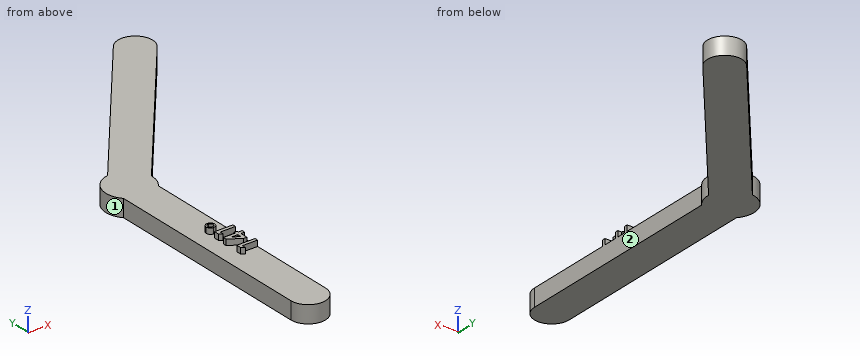
```python
from build123d import *

# Parameters (mm, degrees)
BOSS_EXTRUDE1_DEPTH = 3
BOSS_EXTRUDE2_DEPTH = 1


with BuildPart() as part:
    # Sketch2 → Boss-Extrude1 (new body)
    with BuildSketch(Plane.XY):
        with BuildLine():
            Line((-3, -40), (-3, -2.645751311))
            ThreePointArc((-3, -2.645751311), (-3.770565964, 1.335227437), (-0.666412635, 3.94409612))
            Line((-0.666412635, 3.94409612), (22.841377758, 32.973799631))
            ThreePointArc((22.841377758, 32.973799631), (27.060776815, 33.417276343), (27.504253526, 29.197877285))
            Line((27.504253526, 29.197877285), (3.996463134, 0.168173773))
            ThreePointArc((3.996463134, 0.168173773), (3.770565964, -1.335227437), (3, -2.645751311))
            Line((3, -2.645751311), (3, -40))
            ThreePointArc((3, -40), (0, -43), (-3, -40))
        make_face()
    extrude(amount=BOSS_EXTRUDE1_DEPTH)

    # Sketch3 → Boss-Extrude2 (add)
    # profile 1 of 4: a face of its own
    with BuildSketch(Plane.XY.offset(3)):
        Polygon((-0.175, -25.154881865), (-0.175, -24.27399745), (3, -24.27399745), (3, -24.843869245), (0.354166667, -24.843869245), (0.354166667, -25.495151297), align=None)
    # profile 2 of 4: a face of its own
    with BuildSketch(Plane.XY.offset(3)):
        Polygon((-0.256410256, -21.977973813), (-0.256410256, -21.383933348), (1.819551282, -21.383933348), (1.819551282, -21.09899745), (2.348717949, -21.09899745), (2.348717949, -21.383933348), (3, -21.383933348), (3, -21.953805143), (2.348717949, -21.953805143), (2.348717949, -23.297074373), (1.77184996, -23.297074373), align=None)
        Polygon((1.819551282, -21.953805143), (0.738957332, -21.953805143), (1.819551282, -22.656604622), align=None, mode=Mode.SUBTRACT)
    # profile 3 of 4: a face of its own
    with BuildSketch(Plane.XY.offset(3)):
        Polygon((-0.175, -20.188856224), (-0.175, -19.307971809), (3, -19.307971809), (3, -19.877843604), (0.354166667, -19.877843604), (0.354166667, -20.529125656), align=None)
    # profile 4 of 4: a face of its own
    with BuildSketch(Plane.XY.offset(3)):
        with BuildLine():
            add(Edge.make_bspline(
                [(0.476282051, -16.824958989), (0.501543872, -16.825505484), (0.55122174, -16.826580176), (0.624352745, -16.837013476), (0.694208258, -16.854492691), (0.761803607, -16.876903338), (0.825395964, -16.908042089), (0.886396731, -16.944903837), (0.943669883, -16.989402672), (0.9978957, -17.039014969), (1.047295391, -17.093515132), (1.090947065, -17.151405488), (1.127096601, -17.212864468), (1.157366856, -17.276577248), (1.180332148, -17.343408663), (1.196689885, -17.412864586), (1.20741609, -17.485236986), (1.208449037, -17.534503871), (1.208974359, -17.559559349)],
                knots=[0, 0, 0, 0, 1.048753193, 2.062393874, 3.059725798, 4.03711221, 5.013824111, 5.993903926, 6.992478922, 8.020738441, 9.043061753, 10.043343452, 11.026424807, 11.999358773, 12.968420071, 13.955122655, 14.960044262, 16, 16, 16, 16], degree=3))
            add(Edge.make_bspline(
                [(1.208974359, -17.559559349), (1.208454225, -17.584616682), (1.207431478, -17.633887214), (1.196631189, -17.706233128), (1.180530583, -17.775855144), (1.156529218, -17.842391691), (1.126678292, -17.90615653), (1.090260147, -17.967072817), (1.046482503, -18.024600993), (0.996781055, -18.078582797), (0.942375086, -18.128107638), (0.88420218, -18.171482912), (0.823225465, -18.208946116), (0.758107997, -18.237837437), (0.69067286, -18.261947038), (0.619758864, -18.27798784), (0.545943315, -18.288833106), (0.495615647, -18.289833085), (0.469921875, -18.290343604)],
                knots=[0, 0, 0, 0, 1.037227242, 2.039512271, 3.023626077, 3.993053151, 4.963434463, 5.936395473, 6.927031705, 7.952593414, 8.972234493, 9.969891786, 10.954906455, 11.929570282, 12.915563215, 13.916770353, 14.936449251, 16, 16, 16, 16], degree=3))
            add(Edge.make_bspline(
                [(0.469921875, -18.290343604), (0.445290866, -18.289811451), (0.396869022, -18.288765297), (0.325492116, -18.278103661), (0.256787066, -18.261182775), (0.190979117, -18.23681523), (0.128167681, -18.205730248), (0.067236284, -18.169180135), (0.010175979, -18.123937412), (-0.044275745, -18.073515722), (-0.093962638, -18.018218509), (-0.137555056, -17.95952238), (-0.173973759, -17.89802202), (-0.203993097, -17.834134423), (-0.227847104, -17.767768562), (-0.244158222, -17.698411219), (-0.254789074, -17.626671533), (-0.255866772, -17.577830012), (-0.256410256, -17.553199173)],
                knots=[0, 0, 0, 0, 1.027628768, 2.020204677, 3.0054932, 3.977172113, 4.942988595, 5.928118098, 6.937247537, 7.976812879, 9.023474825, 10.036014018, 11.024160528, 12.002107364, 12.979092523, 13.962271943, 14.972371232, 16, 16, 16, 16], degree=3))
            add(Edge.make_bspline(
                [(-0.256410256, -17.553199173), (-0.255881051, -17.528566172), (-0.254836181, -17.479930408), (-0.244068832, -17.408427146), (-0.227959354, -17.339440503), (-0.203981879, -17.27352423), (-0.173948227, -17.210285117), (-0.137706982, -17.149501332), (-0.093944483, -17.091941849), (-0.043999627, -17.038019265), (0.009956511, -16.987787182), (0.068273488, -16.944627592), (0.128824771, -16.907104674), (0.192846684, -16.877455064), (0.259342082, -16.853394895), (0.329176204, -16.837233977), (0.401748506, -16.826543556), (0.451226198, -16.825491671), (0.476282051, -16.824958989)],
                knots=[0, 0, 0, 0, 1.02774298, 2.029191086, 3.012479778, 3.981238486, 4.951290381, 5.931946007, 6.930416638, 7.964088953, 8.997761269, 10.003308488, 10.98854748, 11.966603007, 12.943696749, 13.935593372, 14.954569896, 16, 16, 16, 16], degree=3))
        make_face()
        with BuildLine():
            add(Edge.make_bspline(
                [(0.479462139, -17.069189758), (0.462471258, -17.069424264), (0.428972226, -17.069886612), (0.379883793, -17.077505977), (0.332524379, -17.088023775), (0.287283463, -17.10328392), (0.24427911, -17.123234284), (0.203398935, -17.147571829), (0.164484674, -17.176174899), (0.128492582, -17.209237523), (0.095853701, -17.245103846), (0.066652511, -17.282897251), (0.042455186, -17.323086522), (0.023016589, -17.365273093), (0.006315159, -17.408801858), (-0.003707976, -17.454711924), (-0.01154919, -17.502263298), (-0.011966436, -17.534718897), (-0.012179487, -17.55129112)],
                knots=[0, 0, 0, 0, 1.061159961, 2.092171217, 3.098605391, 4.092036902, 5.070589041, 6.057187883, 7.061962211, 8.084674938, 9.107387665, 10.090954379, 11.06617917, 12.032717429, 12.99305519, 13.973669989, 14.965331307, 16, 16, 16, 16], degree=3))
            add(Edge.make_bspline(
                [(-0.012179487, -17.55129112), (-0.01157068, -17.568051412), (-0.01036426, -17.601263796), (-0.004409395, -17.650200831), (0.007572839, -17.69685371), (0.022606002, -17.742054962), (0.043122897, -17.784898142), (0.067542797, -17.826391236), (0.096744971, -17.865435361), (0.129769422, -17.902214665), (0.165718261, -17.935960463), (0.204573602, -17.964950546), (0.244977971, -17.990352408), (0.287582445, -18.010455361), (0.331832846, -18.026567734), (0.377821945, -18.038209426), (0.425871214, -18.044356322), (0.458458137, -18.045521173), (0.475010016, -18.046112835)],
                knots=[0, 0, 0, 0, 1.042034071, 2.064906527, 3.055369705, 4.030203466, 5.020228521, 6.000742353, 7.017744738, 8.043920206, 9.069249762, 10.075703201, 11.051782302, 12.029903876, 12.99669358, 13.974371501, 14.971122288, 16, 16, 16, 16], degree=3))
            add(Edge.make_bspline(
                [(0.475010016, -18.046112835), (0.491349767, -18.045520146), (0.523514051, -18.044353455), (0.570936909, -18.038223162), (0.616468237, -18.026465839), (0.660506807, -18.010425399), (0.703332854, -17.990458383), (0.743356347, -17.964229259), (0.782721478, -17.935019181), (0.819574977, -17.900938323), (0.853594861, -17.864058718), (0.883277913, -17.824563201), (0.908722399, -17.783622403), (0.929101491, -17.740636346), (0.945194342, -17.696373754), (0.956841315, -17.650387952), (0.962986781, -17.60233779), (0.964151827, -17.56975099), (0.96474359, -17.553199173)],
                knots=[0, 0, 0, 0, 1.017878107, 2.003660885, 2.970612419, 3.939454555, 4.919652619, 5.904816436, 6.913406512, 7.969270601, 9.02513469, 10.033724766, 11.041277553, 12.021475617, 12.990317753, 13.970071221, 14.968938047, 16, 16, 16, 16], degree=3))
            add(Edge.make_bspline(
                [(0.96474359, -17.553199173), (0.964515736, -17.536840687), (0.964066668, -17.504600367), (0.956359019, -17.457448889), (0.946146284, -17.411789288), (0.929505189, -17.368485652), (0.910263551, -17.326033898), (0.884925795, -17.286252494), (0.856415485, -17.247396305), (0.822504018, -17.212069657), (0.787116244, -17.177952839), (0.747777121, -17.149765554), (0.707718654, -17.124520148), (0.665616684, -17.10387006), (0.621397497, -17.089062601), (0.575848465, -17.07693948), (0.528165265, -17.071009446), (0.49579822, -17.069800121), (0.479462139, -17.069189758)],
                knots=[0, 0, 0, 0, 1.029744634, 2.029484694, 3.00508751, 3.97324883, 4.947661161, 5.937798898, 6.940036528, 7.980134083, 9.020231638, 10.033191535, 11.023329272, 12.003497406, 12.979740652, 13.958541426, 14.969648588, 16, 16, 16, 16], degree=3))
        make_face(mode=Mode.SUBTRACT)
    extrude(amount=BOSS_EXTRUDE2_DEPTH)


solid = part.part
```
The model under review builds one solid part; all positions refer to its coordinate system, in mm. Face numbers are marked on the shaded views. A direction names the side the tool comes from. Coordinates: 2 decimals unless noted, no trailing zeros. Write each loop counter-clockwise with the first axis right and the second up, starting at its lowest first coordinate (ties: lowest second). Pieces come first, ordered by that corner, then holes.
1) Clearance check with flat-ended pins moving along their axes: pin 1 Ø2 at (y, z) = (-18, 1.5) entering from +X; pin 2 Ø1 at (y, z) = (4.5, 3) entering from +X; pin 3 Ø10 at (x, y) = (6.5, 13) entering from -Z; pin 4 Ø0.8 at (x, z) = (1.5, 3.5) entering from -Y. State where each tip first meets the part, or that it passes through.
2) We need section B-B on y = -28. State the section outline as (x, z) points, then the cut area to 3 significant figures.
3) We need section A-A on z = 0.95. State the section outline as (x, y) points, then the cut area to 3 significant figures.
4) Machinability: for the marked faces 1 and 2, which of the approach directions +Z, -Z, +X, -X, +Y, -Y give a long, thin tool a straight path to every point of the face, cutting with its end or side? Answer none if there is none.
5) We need section C-C on x = 5. State the section outline as (y, z) points, then the cut area to 3 significant figures.
6) To check wall thickness, follow probe 1 along X at (y, z) = (-30, 1.3); probe 2 along Z at (x, y) = (11.5, 15.5); probe 3 along X at (y, z) = (15.5, 0.45). State the ranges of each line that lie inside material, in increasing order.
Answer list:
1. pin 1: stops at x = 3
1. pin 2: stops at x = 7.91
1. pin 3: stops at z = 0
1. pin 4: stops at y = -24.84
2. outline: (-3, 0) - (3, 0) - (3, 3) - (-3, 3) - close
2. area: 18.0 mm2
3. outline: (-3, -40) arc R3 ccw to (3, -40) - (3, -2.65) arc R4 ccw to (4, 0.17) - (27.5, 29.2) arc R3 ccw to (22.84, 32.97) - (-0.67, 3.94) arc R4 ccw to (-3, -2.65) - close
3. area: 516 mm2
4. face 1: +Z, -Z, -X
4. face 2: +Z, -Z, +X, -Y
5. outline: (1.41, 0) - (10.94, 0) - (10.94, 3) - (1.41, 3) - close
5. area: 28.6 mm2
6. probe 1: x = -3 to 3
6. probe 2: z = 0 to 3
6. probe 3: x = 8.69 to 16.41
